```python
from build123d import *

# Parameters (mm, degrees)
CROQUIS1_W              = 35
CROQUIS1_H              = 15
SALIENTE_EXTRUIR1_DEPTH = 2
CROQUIS2_R              = 1.75
CORTAR_EXTRUIR1_DEPTH   = 20.144189719
CROQUIS3_W              = 35
CROQUIS3_H              = 1.732050808
SALIENTE_EXTRUIR2_DEPTH = 15
CORTAR_EXTRUIR2_REACH   = 30.333
CROQUIS4_R              = 1.75


with BuildPart() as part:
    # Croquis1 → Saliente-Extruir1 (new body)
    with BuildSketch(Plane(origin=(0, 0, 0), x_dir=(1, 0, 0), z_dir=(0, 1, 0))):
        Rectangle(CROQUIS1_W, CROQUIS1_H)
    extrude(amount=SALIENTE_EXTRUIR1_DEPTH)

    # Croquis2 → Cortar-Extruir1 (cut, through all)
    with BuildSketch(Plane(origin=(0, 2, 0), x_dir=(1, 0, 0), z_dir=(0, 1, 0))):
        with Locations(Location((-14, 4.5, 0), (0, 0, 270))):
            Circle(CROQUIS2_R)
        with Locations(Location((14, 4.5, 0), (0, 0, 270))):
            Circle(CROQUIS2_R)
    extrude(amount=-CORTAR_EXTRUIR1_DEPTH, mode=Mode.SUBTRACT)

    # Croquis3 → Saliente-Extruir2 (add)
    with BuildSketch(Plane(origin=(0, 3.247595264, 5.625), x_dir=(1, 0, 0), z_dir=(0, 0.500000000000001, 0.866025403784438))):
        with Locations((0, -2.883974596)):
            Rectangle(CROQUIS3_W, CROQUIS3_H)
    extrude(amount=SALIENTE_EXTRUIR2_DEPTH)

    # Croquis4 → Cortar-Extruir2 (cut, up to next)
    with BuildSketch(Plane(origin=(0, -3.247595264, 1.875), x_dir=(1, 0, 0), z_dir=(0, -0.8660254037844382, 0.5000000000000011)), mode=Mode.PRIVATE) as cortar_extruir2_sk1:
        with Locations(Location((0, 13.995190528, 0), (0, 0, 270))):
            Circle(CROQUIS4_R)
    cortar_extruir2_tool1 = extrude(cortar_extruir2_sk1.sketch, amount=-CORTAR_EXTRUIR2_REACH, mode=Mode.PRIVATE) & part.part
    add(cortar_extruir2_tool1.solids().sort_by_distance((0, 3.75, 13.995191))[0], mode=Mode.SUBTRACT)


solid = part.part
```
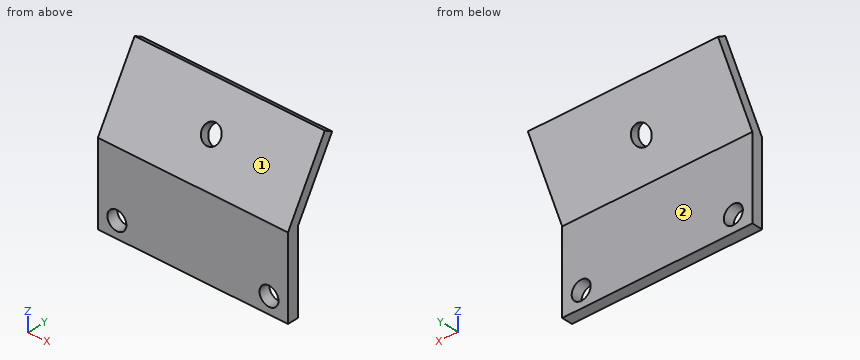
Build history of the part. All positions in model axes, mm. Face numbers are marked on the shaded views. A direction names the side the tool comes from. Give positions to 0.01 mm unless a question says otherwise; leave off trailing zeros. Loops run counter-clockwise (first coordinate to the right, second up) from the corner with the lowest first, then second, coordinate; pieces in that order, holes last.
1) 3-axis set-ups, long thin cutter, end or side, ignore diameter. For the marked faces 1 and 2: which of +Z, -Z, +X, -X, +Y, -Y reach the whole face in a straight line?
Values follow:
face 1: +Z, +X, -X, -Y
face 2: -Z, +X, -X, +Y
2) Band-saw the part on C-C on x = -9. List the corners of the cut face in (y, z), then the cut area to 3 significant figures.
Values follow:
outline: (0, -7.5) - (2, -7.5) - (2, 7.5) - (9, 19.62) - (7.5, 20.49) - (0, 7.5) - close
area: 55.1 mm2
3) Probe line 1 along X through (y, z) = (0.9, -4.5); line 2 along Y through (x, z) = (-12.5, 4); line 3 along Z through (x, y) = (5, 6.5). List the from-to ranges inside material, lowest first.
Values follow:
line 1: x = -17.5 to -15.75, -12.25 to 12.25, 15.75 to 17.5
line 2: y = 0 to 2
line 3: z = 15.29 to 18.76
4) Drop flat-ended pins along their axis: P1, Ø3, axis at x = -0.5, z = 16, coming from the +Y side; P2, Ø1.5, axis at x = -5.5, z = 6, coming from the +Y side; P3, Ø16.5, axis at x = -1, z = 3.5, coming from the +Y side. Give the stop position or say it passes through.
Values follow:
P1: stops at y = 7.77
P2: stops at y = 2
P3: stops at y = 4.45
5) Band-saw the part on A-A on z = -4.5. List the corners of the cut face in (x, y).
Values follow:
outline: (-17.5, 0) - (-15.75, 0) - (-15.75, 2) - (-17.5, 2) - close; (-12.25, 0) - (12.25, 0) - (12.25, 2) - (-12.25, 2) - close; (15.75, 0) - (17.5, 0) - (17.5, 2) - (15.75, 2) - close
6) Band-saw the part on B-B on x = 14. List the corners of the cut face in (y, z), then the cut area to 3 significant figures.
Values follow:
outline: (0, -7.5) - (2, -7.5) - (2, -6.25) - (0, -6.25) - close; (0, -2.75) - (2, -2.75) - (2, 7.5) - (9, 19.62) - (7.5, 20.49) - (0, 7.5) - close
area: 48.1 mm2
7) Band-saw the part on D-D on z = 10.5. List the corners of the cut face in (x, y).
Values follow:
outline: (-17.5, 1.73) - (17.5, 1.73) - (17.5, 3.73) - (-17.5, 3.73) - close
